Job drawing, mm, ordinate dimensions from the low corner. One solid piece. Round coordinates to 2 decimals unless told otherwise and drop trailing zeros. Order: outer loops, then holes, each group sorted by start corner. A loop starts at its lowest first (then second) coordinate and runs counter-clockwise, first axis right, second up. Notation, with made-up numbers: (-25, 85.25) -> (10, 85.25) arc R19 ccw to (10, 103.25) -> close; hole circle Ø5 at (28, -3). An arc over 180 degrees is marked (long way). Use CSV: the item, a comma, the result in double quotes.
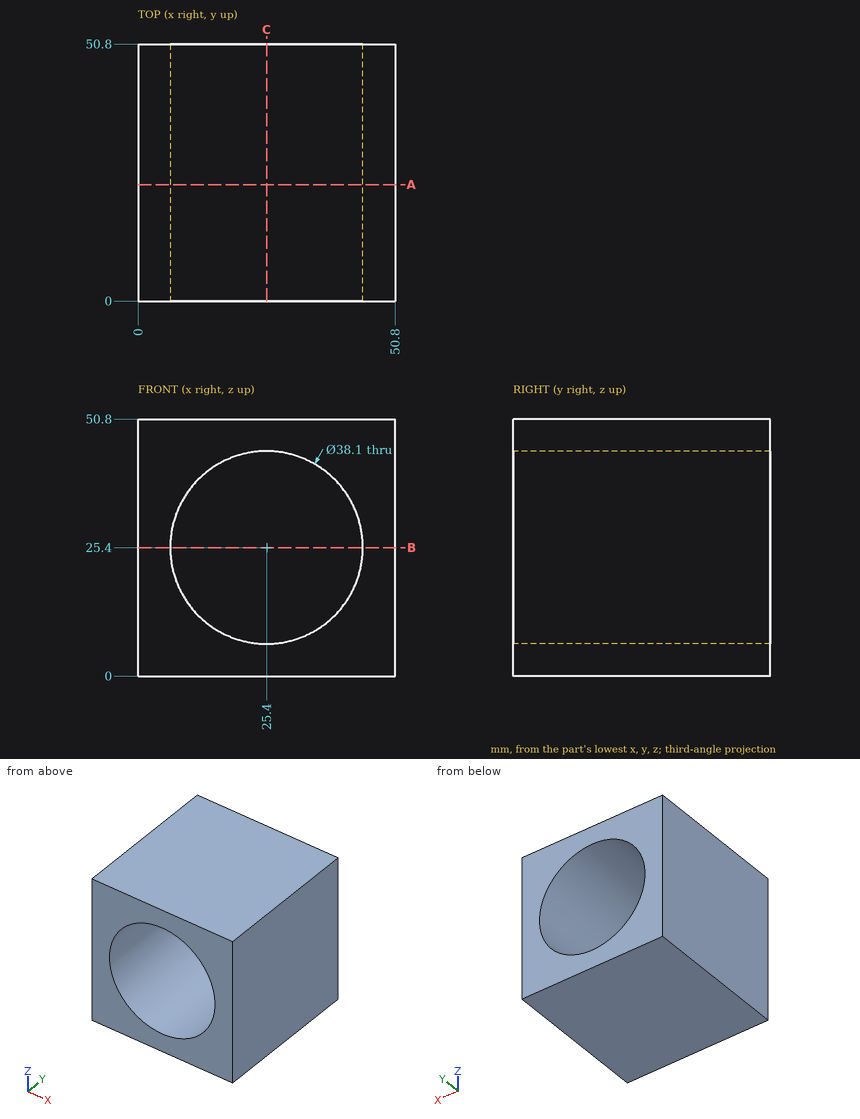
(1) Cut at B-B, the plane z = 25.4. Give the cut face in (x, y), then the cut area to 3 significant figures.
Reply:
outline,"(0, 0) -> (6.35, 0) -> (6.35, 50.8) -> (0, 50.8) -> close; (44.45, 0) -> (50.8, 0) -> (50.8, 50.8) -> (44.45, 50.8) -> close"
area,"645 mm2"
(2) Probe probe 1 along X at (y, z) = (16, 25); probe 2 along Z at (x, y) = (26, 35); probe 3 along Z at (x, y) = (22, 9). List the from-to ranges inside material, lowest first. Write a range as [from, to].
Reply:
probe 1,"[0, 6.35], [44.45, 50.8]"
probe 2,"[0, 6.36], [44.44, 50.8]"
probe 3,"[0, 6.66], [44.14, 50.8]"
(3) Cut at A-A, the plane y = 23. Give the cut face in (x, z).
Reply:
outline,"(0, 0) -> (50.8, 0) -> (50.8, 50.8) -> (0, 50.8) -> close; hole circle Ø38.1 at (25.4, 25.4)"
(4) Cut at C-C, the plane x = 25.4. Give the cut face in (y, z), then the cut area to 3 significant figures.
Reply:
outline,"(0, 0) -> (50.8, 0) -> (50.8, 6.35) -> (0, 6.35) -> close; (0, 44.45) -> (50.8, 44.45) -> (50.8, 50.8) -> (0, 50.8) -> close"
area,"645 mm2"
